```python
from build123d import *

# Parameters (mm, degrees)
EXTRUDE_THIN1_DEPTH    = 756.30962295
SKETCH2_R              = 40
EXTRUDE1_DEPTH         = 3
LPATTERN1_COUNT        = 7
LPATTERN1_PITCH        = 115
LPATTERN2_COUNT        = 7
LPATTERN2_PITCH        = 115
F_10_CLEARANCE_HOLE1_D = 4.9784


with BuildPart() as part:
    # Sketch1 → Extrude-Thin1 (new body, symmetric)
    with BuildSketch(Plane.XY):
        with BuildLine():
            Line((25.4, 49), (2.54, 49))
            ThreePointArc((2.54, 49), (0.743948776, 48.256051224), (0, 46.46))
            Line((0, 46.46), (0, -46.46))
            ThreePointArc((0, -46.46), (0.743948776, -48.256051224), (2.54, -49))
            Line((2.54, -49), (25.4, -49))
            Line((25.4, -49), (25.4, -47))
            Line((25.4, -47), (2.54, -47))
            ThreePointArc((2.54, -47), (2.158162338, -46.841837662), (2, -46.46))
            Line((2, -46.46), (2, 46.46))
            ThreePointArc((2, 46.46), (2.158162338, 46.841837662), (2.54, 47))
            Line((2.54, 47), (25.4, 47))
            Line((25.4, 47), (25.4, 49))
        make_face()
    extrude(amount=EXTRUDE_THIN1_DEPTH, both=True)

    # Sketch2 → Extrude1 (cut, through all)
    with BuildSketch(Plane(origin=(2, 0, 0), x_dir=(0, 0, -1), z_dir=(1, 0, 0))):
        Circle(SKETCH2_R)
    extrude1 = extrude(amount=-EXTRUDE1_DEPTH, mode=Mode.SUBTRACT)

    # LPattern1: Extrude1 ×7
    with Locations(*[(0, 0, i * LPATTERN1_PITCH) for i in range(1, LPATTERN1_COUNT)]):
        add(extrude1, mode=Mode.SUBTRACT)

    # LPattern2: Extrude1 ×7
    with Locations(*[(0, 0, -i * LPATTERN2_PITCH) for i in range(1, LPATTERN2_COUNT)]):
        add(extrude1, mode=Mode.SUBTRACT)

    # #10 Clearance Hole1 (through all)
    with Locations(Plane.XZ.offset(49)):
        with Locations((13.97, 744.30962295), (13.97, 714.30962295)):
            f_10_clearance_hole1 = Hole(F_10_CLEARANCE_HOLE1_D / 2)

    # Mirror1: #10 Clearance Hole1 across plane
    add(f_10_clearance_hole1.mirror(Plane.XY), mode=Mode.SUBTRACT)


solid = part.part
```
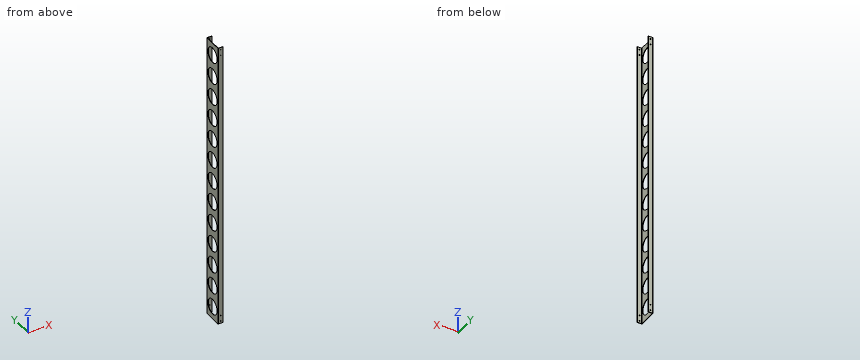
Part model, mm, in its own coordinate system. Round coordinates to 2 decimals unless told otherwise and drop trailing zeros. Write each loop counter-clockwise with the first axis right and the second up, starting at its lowest first coordinate (ties: lowest second). Pieces come first, ordered by that corner, then holes. Notation, with made-up numbers: (56, 53.5) -> (60, 53.5) arc R13 cw to (60, 62.5) -> close; hole circle Ø2 at (36, -31.75). An arc over 180 degrees is marked (long way). Return JSON: item names as keys, results as strings. Group by question number.
Q1. Probe L1, parallel to Z at x = 13.97, y = 48.55; L2, parallel to Y at x = 6.75, z = 694; L3, parallel to X at y = 43, z = -133. List the from-to ranges inside material, lowest first. Write a range as [from, to].
Q2. Saw through at A-A on z = 460. Write the cut outline in (x, y), plus the area to 3 significant figures.
Q3. Saw through at C-C on z = 239. Write the cut outline in (x, y).
Q4. Saw through at B-B on y = 0. State how many separate pieces and enclosed holes the cut face has, plus the area to 3 significant figures.
Q5. Pin check, flat tips, straight feed: pin 1 (8 mm diameter, centred on y = 36, z = 526.5, fed in from +X); pin 2 (4 mm diameter, centred on x = 13.97, z = -744.31, fed in from -Y). Stop position of each tip, or through.
Answer:
{
 "1": {"L1": "[-756.31, -746.8], [-741.82, -716.8], [-711.82, 711.82], [716.8, 741.82], [746.8, 756.31]", "L2": "[-49, -47], [47, 49]", "L3": "[0, 2]"},
 "2": {"outline": "(0, -46.46) arc R2.54 ccw to (2.54, -49) -> (25.4, -49) -> (25.4, -47) -> (2.54, -47) arc R0.54 cw to (2, -46.46) -> (2, -40) -> (0, -40) -> close; (0, 40) -> (2, 40) -> (2, 46.46) arc R0.54 cw to (2.54, 47) -> (25.4, 47) -> (25.4, 49) -> (2.54, 49) arc R2.54 ccw to (0, 46.46) -> close", "area": "127 mm2"},
 "3": {"outline": "(0, -46.46) arc R2.54 ccw to (2.54, -49) -> (25.4, -49) -> (25.4, -47) -> (2.54, -47) arc R0.54 cw to (2, -46.46) -> (2, -38.97) -> (0, -38.97) -> close; (0, 38.97) -> (2, 38.97) -> (2, 46.46) arc R0.54 cw to (2.54, 47) -> (25.4, 47) -> (25.4, 49) -> (2.54, 49) arc R2.54 ccw to (0, 46.46) -> close"},
 "4": {"separate pieces": "14", "enclosed holes": "0", "area": "945 mm2"},
 "5": {"pin 1": "x = 2", "pin 2": "through"}
}
